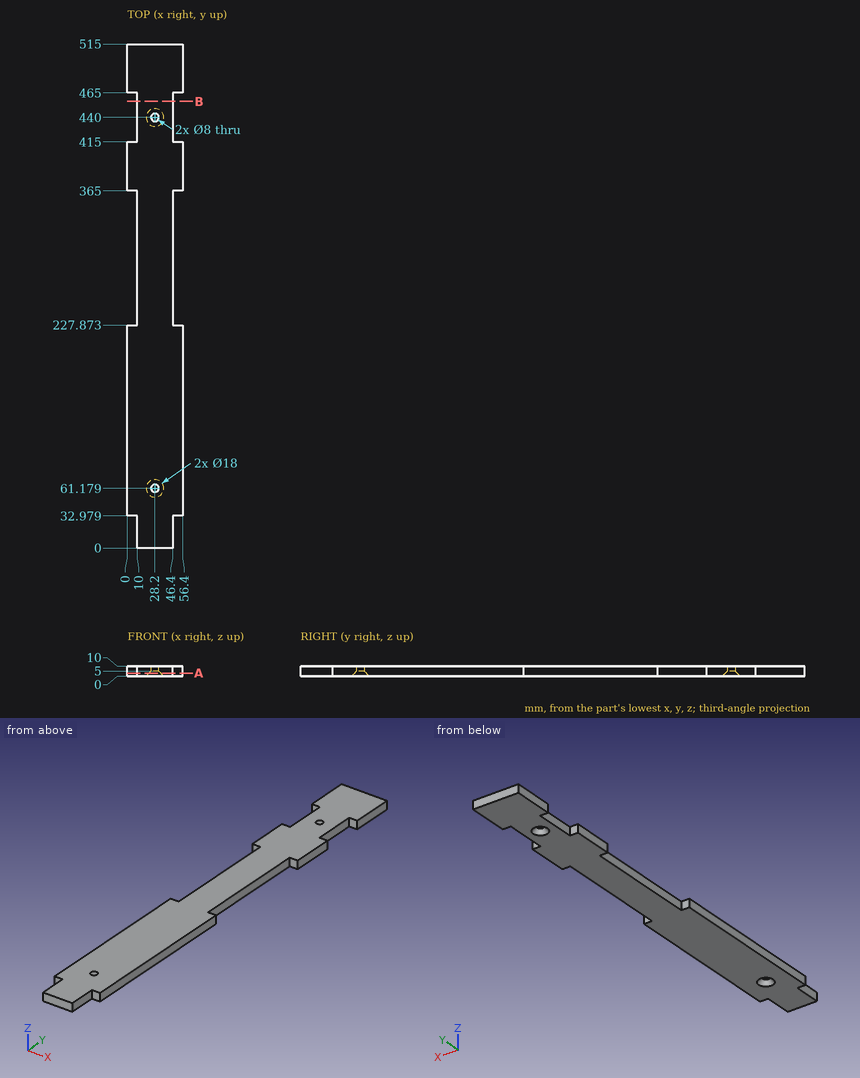
Here's the drawing with two shaded views (mm, measured from the low corner). I have some questions. Round coordinates to 2 decimals unless told otherwise and drop trailing zeros. Loops run counter-clockwise (first coordinate to the right, second up) from the corner with the lowest first, then second, coordinate; pieces in that order, holes last.
1. If I drill on probe 1 along Y at (x, z) = (28.2, 6.7); probe 2 along Y at (x, z) = (50, 5); probe 3 along X at (y, z) = (464, 1), over which ranges is the centre line in solid material (lowest first)?
Answers:
probe 1: y = 0 to 57.18, 65.18 to 436, 444 to 515
probe 2: y = 32.98 to 227.87, 365 to 415, 465 to 515
probe 3: x = 10 to 46.4
2. Suppose I cut it at A-A, the plane z = 3. Please give me the cut outline in (x, y), and give its area (3 significant figures).
Answers:
outline: (0, 32.98) - (10, 32.98) - (10, 0) - (46.4, 0) - (46.4, 32.98) - (56.4, 32.98) - (56.4, 227.87) - (46.4, 227.87) - (46.4, 365) - (56.4, 365) - (56.4, 415) - (46.4, 415) - (46.4, 465) - (56.4, 465) - (56.4, 515) - (0, 515) - (0, 465) - (10, 465) - (10, 415) - (0, 415) - (0, 365) - (10, 365) - (10, 227.87) - (0, 227.87) - close; hole circle Ø12 at (28.2, 61.18); hole circle Ø12 at (28.2, 440)
area: 24,400 mm2
3. Suppose I cut it at B-B, the plane y = 456.5. Please give me the cut outline in (x, z).
Answers:
outline: (10, 0) - (46.4, 0) - (46.4, 10) - (10, 10) - close
4. Will these pins go through, and if not, where does the flat tip stop? pin 1 (1 mm diameter, centred on x = 28.5, z = 3.5, fed in from -Y); pin 2 (5 mm diameter, centred on y = 306, z = 4, fed in from -X); pin 3 (5 mm diameter, centred on x = 49.5, z = 6, fed in from -Y); pin 4 (7 mm diameter, centred on x = 28.2, y = 440, fed in from +Z).
Answers:
pin 1: stops at y = 0
pin 2: stops at x = 10
pin 3: stops at y = 32.98
pin 4: passes through
